Design review of the part built by this model. Coordinates are the model's own, in mm. A direction names the side the tool comes from. Give positions to 0.01 mm unless a question says otherwise; leave off trailing zeros. Write each loop counter-clockwise with the first axis right and the second up, starting at its lowest first coordinate (ties: lowest second). Pieces come first, ordered by that corner, then holes.
```python
from build123d import *

# Parameters (mm, degrees)
SKETCH1_W            = 87
SKETCH1_H            = 60
BOSS_EXTRUDE1_DEPTH  = 20
SKETCH2_R            = 22.5
CUT_EXTRUDE1_DEPTH   = 20
SKETCH3_W            = 82
SKETCH3_H            = 55
CUT_EXTRUDE2_DEPTH   = 16
SKETCH4_W            = 6.45
SKETCH4_H            = 23.85
BOSS_EXTRUDE2_DEPTH  = 3
SKETCH5_W            = 2.45
SKETCH5_H            = 19
BOSS_EXTRUDE3_DEPTH  = 2
FILLET5_R            = 3
FILLET7_R            = 2
SKETCH6_W            = 2.45
SKETCH6_H            = 19
BOSS_EXTRUDE4_DEPTH  = 2
FILLET8_R            = 3
FILLET9_R            = 2
SKETCH7_W            = 6.45
SKETCH7_H            = 3
BOSS_EXTRUDE5_DEPTH  = 2.5
SKETCH9_W            = 6.45
SKETCH9_H            = 3
BOSS_EXTRUDE6_DEPTH  = 2.5
CUT_EXTRUDE3_DEPTH   = 81.731271908
SKETCH46_W           = 6.45
SKETCH46_H           = 23.85
BOSS_EXTRUDE22_DEPTH = 3
SKETCH47_W           = 2.45
SKETCH47_H           = 19
BOSS_EXTRUDE23_DEPTH = 2
SKETCH48_W           = 2.45
SKETCH48_H           = 19
BOSS_EXTRUDE24_DEPTH = 2
FILLET11_R           = 3
FILLET12_R           = 3
FILLET13_R           = 2
FILLET14_R           = 2
SKETCH49_W           = 6.45
SKETCH49_H           = 3
BOSS_EXTRUDE25_DEPTH = 2.5
SKETCH50_W           = 6.45
SKETCH50_H           = 3
BOSS_EXTRUDE26_DEPTH = 2.5
CUT_EXTRUDE8_DEPTH   = 81.731271908


with BuildPart() as part:
    # Sketch1 → Boss-Extrude1 (new body)
    with BuildSketch(Plane(origin=(0, 0, 0), x_dir=(1, 0, 0), z_dir=(0, 1, 0))):
        with Locations((-17.058139535, -0.906976744)):
            Rectangle(SKETCH1_W, SKETCH1_H)
    extrude(amount=BOSS_EXTRUDE1_DEPTH)

    # Sketch2 → Cut-Extrude1 (cut)
    with BuildSketch(Plane(origin=(0, 20, 0), x_dir=(1, 0, 0), z_dir=(0, 1, 0))):
        with Locations(Location((-17.058139535, -0.906976744, 0), (0, 0, 270))):
            Circle(SKETCH2_R)
    extrude(amount=-CUT_EXTRUDE1_DEPTH, mode=Mode.SUBTRACT)

    # Sketch3 → Cut-Extrude2 (cut)
    with BuildSketch(Plane.XZ):
        with Locations((-17.058139535, 0.906976744)):
            Rectangle(SKETCH3_W, SKETCH3_H)
    extrude(amount=-CUT_EXTRUDE2_DEPTH, mode=Mode.SUBTRACT)

    # Sketch4 → Boss-Extrude2 (add)
    with BuildSketch(Plane.ZY.offset(-23.941860465)):
        with Locations((-15.368023256, 4.075)):
            Rectangle(SKETCH4_W, SKETCH4_H)
        with Locations((17.181976744, 4.075)):
            Rectangle(SKETCH4_W, SKETCH4_H)
    extrude(amount=BOSS_EXTRUDE2_DEPTH)

    # Sketch5 → Boss-Extrude3 (add)
    with BuildSketch(Plane.ZY.offset(-20.941860465)):
        with Locations((-15.368023256, 1.65)):
            Rectangle(SKETCH5_W, SKETCH5_H)
    extrude(amount=BOSS_EXTRUDE3_DEPTH)

    # Fillet5
    fillet5_edges = [part.edges().sort_by_distance(p)[0] for p in [
        (18.941860465, -7.85, -15.368023256),
    ]]
    fillet(fillet5_edges, radius=FILLET5_R)

    # Fillet7
    fillet7_edges = [part.edges().sort_by_distance(p)[0] for p in [
        (18.941860465, 11.15, -15.368023256),
    ]]
    fillet(fillet7_edges, radius=FILLET7_R - 0.0001)  # a hair under: the kernel refuses the full size

    # Sketch6 → Boss-Extrude4 (add)
    with BuildSketch(Plane.ZY.offset(-20.941860465)):
        with Locations((17.181976744, 1.65)):
            Rectangle(SKETCH6_W, SKETCH6_H)
    extrude(amount=BOSS_EXTRUDE4_DEPTH)

    # Fillet8
    fillet8_edges = [part.edges().sort_by_distance(p)[0] for p in [
        (18.941860465, -7.85, 17.181976744),
    ]]
    fillet(fillet8_edges, radius=FILLET8_R)

    # Fillet9
    fillet9_edges = [part.edges().sort_by_distance(p)[0] for p in [
        (18.941860465, 11.15, 17.181976744),
    ]]
    fillet(fillet9_edges, radius=FILLET9_R - 0.0001)  # a hair under: the kernel refuses the full size

    # Sketch7 → Boss-Extrude5 (add)
    with BuildSketch(Plane(origin=(23.941860465, 0, 0), x_dir=(0, 0, -1), z_dir=(1, 0, 0))):
        with Locations((-17.181976744, -6.35)):
            Rectangle(SKETCH7_W, SKETCH7_H)
    extrude(amount=BOSS_EXTRUDE5_DEPTH)

    # Sketch9 → Boss-Extrude6 (add)
    with BuildSketch(Plane(origin=(23.941860465, 0, 0), x_dir=(0, 0, -1), z_dir=(1, 0, 0))):
        with Locations((15.368023256, -6.35)):
            Rectangle(SKETCH9_W, SKETCH9_H)
    extrude(amount=BOSS_EXTRUDE6_DEPTH)

    # Sketch8 → Cut-Extrude3 (cut, through all)
    with BuildSketch(Plane.XY.offset(20.406976744)):
        Polygon((26.441860465, -5.85), (24.191860465, -7.85), (26.441860465, -7.85), align=None)
    extrude(amount=-CUT_EXTRUDE3_DEPTH, mode=Mode.SUBTRACT)

    # Sketch46 → Boss-Extrude22 (add)
    with BuildSketch(Plane(origin=(-58.058139535, 0, 0), x_dir=(0, 0, -1), z_dir=(1, 0, 0))):
        with Locations((-17.181976744, 4.075)):
            Rectangle(SKETCH46_W, SKETCH46_H)
        with Locations((15.368023256, 4.075)):
            Rectangle(SKETCH46_W, SKETCH46_H)
    extrude(amount=BOSS_EXTRUDE22_DEPTH)

    # Sketch47 → Boss-Extrude23 (add)
    with BuildSketch(Plane(origin=(-55.058139535, 0, 0), x_dir=(0, 0, -1), z_dir=(1, 0, 0))):
        with Locations((-17.181976744, 1.65)):
            Rectangle(SKETCH47_W, SKETCH47_H)
    extrude(amount=BOSS_EXTRUDE23_DEPTH)

    # Sketch48 → Boss-Extrude24 (add)
    with BuildSketch(Plane(origin=(-55.058139535, 0, 0), x_dir=(0, 0, -1), z_dir=(1, 0, 0))):
        with Locations((15.368023256, 1.65)):
            Rectangle(SKETCH48_W, SKETCH48_H)
    extrude(amount=BOSS_EXTRUDE24_DEPTH)

    # Fillet11
    fillet11_edges = [part.edges().sort_by_distance(p)[0] for p in [
        (-53.058139535, -7.85, 17.181976744),
    ]]
    fillet(fillet11_edges, radius=FILLET11_R)

    # Fillet12
    fillet12_edges = [part.edges().sort_by_distance(p)[0] for p in [
        (-53.058139535, -7.85, -15.368023256),
    ]]
    fillet(fillet12_edges, radius=FILLET12_R)

    # Fillet13
    fillet13_edges = [part.edges().sort_by_distance(p)[0] for p in [
        (-53.058139535, 11.15, -15.368023256),
    ]]
    fillet(fillet13_edges, radius=FILLET13_R - 0.0001)  # a hair under: the kernel refuses the full size

    # Fillet14
    fillet14_edges = [part.edges().sort_by_distance(p)[0] for p in [
        (-53.058139535, 11.15, 17.181976744),
    ]]
    fillet(fillet14_edges, radius=FILLET14_R - 0.0001)  # a hair under: the kernel refuses the full size

    # Sketch49 → Boss-Extrude25 (add)
    with BuildSketch(Plane.ZY.offset(58.058139535)):
        with Locations((17.181976744, -6.35)):
            Rectangle(SKETCH49_W, SKETCH49_H)
    extrude(amount=BOSS_EXTRUDE25_DEPTH)

    # Sketch50 → Boss-Extrude26 (add)
    with BuildSketch(Plane.ZY.offset(58.058139535)):
        with Locations((-15.368023256, -6.35)):
            Rectangle(SKETCH50_W, SKETCH50_H)
    extrude(amount=BOSS_EXTRUDE26_DEPTH)

    # Sketch52 → Cut-Extrude8 (cut, through all)
    with BuildSketch(Plane(origin=(0, 0, -18.593023256), x_dir=(-1, 0, 0), z_dir=(0, 0, -1))):
        Polygon((60.558139535, -5.85), (58.308139535, -7.85), (60.558139535, -7.85), align=None)
    extrude(amount=-CUT_EXTRUDE8_DEPTH, mode=Mode.SUBTRACT)


solid = part.part
```
(1) Tool access review of faces 1 (the face through (-57, 4, -18.593)), 2 (the face through (25, -4.85, 17)), 3 (the face through (-54.365, -7.326, 17.137)), 4 (the face through (-58.058, -2, 17)): name each direction out of +Z, -Z, +X, -X, +Y, -Y from which nothing blocks a thin tool from reaching the whole face with its end or side.
Resolved:
face 1: -Y
face 2: +Z, -Z, +X
face 3: +Z, -Z, -Y
face 4: +Z, -Z, -X
(2) To check wall thickness, follow L1, parallel to X at y = 8.75, z = 22; L2, parallel to Z at x = -52, y = 14.25; L3, parallel to X at y = 14, z = -13. State the ranges of each line that lie inside material, in increasing order.
Resolved:
L1: x = -60.56 to -58.06, 23.94 to 26.44
L2: z = -29.09 to -26.59, 28.41 to 30.91
L3: x = -60.56 to -55.06, 20.94 to 26.44
(3) Clearance check with flat-ended pins moving along their axes: P1, Ø8, axis at x = -43, z = -21, coming from the -Y side; P2, Ø0.6, axis at x = -54.5, y = -0.5, coming from the +Z side; P3, Ø2.5, axis at y = -2, z = -16.5, coming from the -X side. State where each tip first meets the part, or that it passes through.
Resolved:
P1: stops at y = 16
P2: stops at z = 18.41
P3: stops at x = -58.06
(4) Consider section A-A, the plane z = -20. Give the boundary of the cut face in (x, y), then the cut area to 3 significant figures.
Resolved:
outline: (-60.56, 0) - (-58.06, 0) - (-58.06, 16) - (-25.37, 16) - (-25.37, 20) - (-60.56, 20) - close; (-8.74, 16) - (23.94, 16) - (23.94, 0) - (26.44, 0) - (26.44, 20) - (-8.74, 20) - close
area: 361 mm2
(5) Consider section C-C, the plane y = 13.75. Give the boundary of the cut face in (x, z), then the cut area to 3 significant figures.
Resolved:
outline: (-60.56, -29.09) - (26.44, -29.09) - (26.44, 30.91) - (-60.56, 30.91) - close; hole (-58.06, -26.59) - (23.94, -26.59) - (23.94, -18.59) - (20.94, -18.59) - (20.94, -12.14) - (23.94, -12.14) - (23.94, 13.96) - (20.94, 13.96) - (20.94, 20.41) - (23.94, 20.41) - (23.94, 28.41) - (-58.06, 28.41) - (-58.06, 20.41) - (-55.06, 20.41) - (-55.06, 13.96) - (-58.06, 13.96) - (-58.06, -12.14) - (-55.06, -12.14) - (-55.06, -18.59) - (-58.06, -18.59) - close
area: 787 mm2
(6) Mouldability with a two-part tool opening along Y and no side actions: class faces 5 (the face through (20.248, -7.326, 17.227)), 6 (the face through (-58.058, -2, -15)), 7 (the face through (-58.058, 8, 1)) as pulls with the +Y half, pulls with the -Y half, needs draft (parallel to the pull), parting line crosses it, or undercut.
Resolved:
face 5: pulls with the -Y half
face 6: undercut
face 7: needs draft
(7) Consider section B-B, the plane x = -22.5. Give the boundary of the cut face in (y, z).
Resolved:
outline: (0, -29.09) - (20, -29.09) - (20, -20.93) - (16, -20.93) - (16, -26.59) - (0, -26.59) - close; (0, 28.41) - (16, 28.41) - (16, 22.74) - (20, 22.74) - (20, 30.91) - (0, 30.91) - close
(8) Consider section D-D, the plane x = 8.5. Give the boundary of the cut face in (y, z), then the cut area to 3 significant figures.
Resolved:
outline: (0, -29.09) - (20, -29.09) - (20, 30.91) - (0, 30.91) - (0, 28.41) - (16, 28.41) - (16, -26.59) - (0, -26.59) - close
area: 320 mm2
